from build123d import *

# Parameters (mm, degrees)
BOSS_EXTRUDE1_DEPTH = 53.975
CUT_EXTRUDE1_DEPTH  = 140.411114894
CUT_EXTRUDE2_DEPTH  = 3.175
BOSS_EXTRUDE2_DEPTH = 15.875
CUT_EXTRUDE3_DEPTH  = 12.7
CHAMFER1_SIZE       = 1.651
CUT_EXTRUDE4_DEPTH  = 12.7
FILLET1_R           = 12.7
SKETCH9_R           = 6.35
CUT_EXTRUDE5_DEPTH  = 12.7
SKETCH10_R          = 9.525
CUT_EXTRUDE6_DEPTH  = 3.175
SKETCH11_R          = 13.97
BOSS_EXTRUDE3_DEPTH = 4.1275
SKETCH12_R          = 11.43
CUT_EXTRUDE7_DEPTH  = 124.457441957
SKETCH13_W          = 29.21
SKETCH13_H          = 6.35
BOSS_EXTRUDE4_DEPTH = 17.78
CUT_EXTRUDE8_DEPTH  = 131.033845412
FILLET3_R           = 1.905
FILLET4_R           = 1.27


with BuildPart() as part:
    # Sketch1 → Boss-Extrude1 (new, symmetric)
    with BuildSketch(Plane.XY):
        with BuildLine():
            Line((0, 0), (0, 12.7))
            Line((0, 12.7), (76.2, 12.7))
            Line((76.2, 12.7), (118.856216575, -29.956216575))
            Line((118.856216575, -29.956216575), (112.57003729, -36.24239586))
            Line((112.57003729, -36.24239586), (91.206616946, -14.878975516))
            ThreePointArc((91.206616946, -14.878975516), (74.725910826, -3.866919748), (55.285592462, 0))
            Line((55.285592462, 0), (0, 0))
        make_face()
    extrude(amount=BOSS_EXTRUDE1_DEPTH, both=True)

    # Sketch2 → Cut-Extrude1 (cut, through all)
    with BuildSketch(Plane(origin=(0, 12.7, 0), x_dir=(1, 0, 0), z_dir=(0, 1, 0))):
        with BuildLine():
            Line((25.4, 53.975), (25.4, 34.925))
            ThreePointArc((25.4, 34.925), (38.1, 22.225), (50.8, 34.925))
            Line((50.8, 34.925), (50.8, 53.975))
            Line((50.8, 53.975), (25.4, 53.975))
        make_face()
        with BuildLine():
            Line((25.4, -53.975), (50.8, -53.975))
            Line((50.8, -53.975), (50.8, -34.925))
            ThreePointArc((50.8, -34.925), (38.1, -22.225), (25.4, -34.925))
            Line((25.4, -34.925), (25.4, -53.975))
        make_face()
    extrude(amount=-CUT_EXTRUDE1_DEPTH, mode=Mode.SUBTRACT)

    # Sketch4 → Cut-Extrude2 (cut, symmetric)
    with BuildSketch(Plane(origin=(0, 6.35, 0), x_dir=(1, 0, 0), z_dir=(0, 1, 0))):
        with BuildLine():
            Line((59.055, -34.925), (59.055, -53.975))
            Line((59.055, -53.975), (17.145, -53.975))
            Line((17.145, -53.975), (17.145, -34.925))
            ThreePointArc((17.145, -34.925), (38.1, -13.97), (59.055, -34.925))
        make_face()
        with BuildLine():
            Line((17.145, 53.975), (17.145, 34.925))
            ThreePointArc((17.145, 34.925), (38.1, 13.97), (59.055, 34.925))
            Line((59.055, 34.925), (59.055, 53.975))
            Line((59.055, 53.975), (17.145, 53.975))
        make_face()
    extrude(amount=CUT_EXTRUDE2_DEPTH, both=True, mode=Mode.SUBTRACT)

    # Sketch5 → Boss-Extrude2 (add, symmetric)
    with BuildSketch(Plane.XY):
        Polygon((0, 12.7), (0, 46.784531851), (76.2, 19.05), (76.2, 12.7), align=None)
    extrude(amount=BOSS_EXTRUDE2_DEPTH, both=True)

    # Sketch6 → Cut-Extrude3 (cut)
    with BuildSketch(Plane(origin=(15.036258699, 41.31178125, 0), x_dir=(0.9396926207859106, -0.3420201433256628, 0), z_dir=(0.3420201433256627, 0.9396926207859105, 0))):
        with BuildLine():
            Line((13.631742372, 3.175), (30.56575305, 3.175))
            ThreePointArc((30.56575305, 3.175), (52.197747711, 0), (30.56575305, -3.175))
            Line((30.56575305, -3.175), (13.631742372, -3.175))
            ThreePointArc((13.631742372, -3.175), (-8.000252289, 0), (13.631742372, 3.175))
        make_face()
    extrude(amount=-CUT_EXTRUDE3_DEPTH, mode=Mode.SUBTRACT)

    # Chamfer1
    chamfer1_edges = [part.edges().sort_by_distance(p)[0] for p in [
        (7.518480659, 44.048028684, 0),
        (35.802288852, 33.75356439, 3.175),
        (64.086097045, 23.459100096, 0),
        (35.802288852, 33.75356439, -3.175),
    ]]
    chamfer(chamfer1_edges, length=CHAMFER1_SIZE)

    # Sketch7 → Cut-Extrude4 (cut)
    with BuildSketch(Plane(origin=(44.45, 44.45, 0), x_dir=(0, 0, -1), z_dir=(0.7071067811865483, 0.7071067811865468, 0))):
        with BuildLine():
            Line((-34.925, -60.776280605), (-53.975, -60.776280605))
            Line((-53.975, -60.776280605), (-53.975, -105.226280605))
            Line((-53.975, -105.226280605), (-8.3e-08, -105.226280605))
            ThreePointArc((-8.3e-08, -105.226280605), (-11.225320181, -100.576600727), (-15.875, -89.351280605))
            Line((-15.875, -89.351280605), (-34.925, -89.351280605))
            Line((-34.925, -89.351280605), (-34.925, -60.776280605))
        make_face()
        with BuildLine():
            ThreePointArc((15.875, -89.351280605), (11.225320122, -100.576600786), (-8.3e-08, -105.226280605))
            Line((-8.3e-08, -105.226280605), (53.975, -105.226280605))
            Line((53.975, -105.226280605), (53.975, -60.776280605))
            Line((53.975, -60.776280605), (34.925, -60.776280605))
            Line((34.925, -60.776280605), (34.925, -89.351280605))
            Line((34.925, -89.351280605), (15.875, -89.351280605))
        make_face()
    extrude(amount=-CUT_EXTRUDE4_DEPTH, mode=Mode.SUBTRACT)

    # Fillet1
    fillet1_edges = [part.edges().sort_by_distance(p)[0] for p in [
        (104.487806781, -21.873986066, 34.925),
        (104.487806781, -21.873986066, -34.925),
        (0, 6.35, 53.975),
        (0, 6.35, -53.975),
    ]]
    fillet(fillet1_edges, radius=FILLET1_R)

    # Sketch9 → Cut-Extrude5 (cut)
    with BuildSketch(Plane(origin=(44.45, 44.45, 0), x_dir=(0, 0, -1), z_dir=(0.7071067811865482, 0.7071067811865468, 0))):
        with Locations(Location((-22.225, -76.651280605, 0), (0, 0, 90))):
            Circle(SKETCH9_R)
        with Locations(Location((22.225, -76.651280605, 0), (0, 0, 90))):
            Circle(SKETCH9_R)
    extrude(amount=-CUT_EXTRUDE5_DEPTH, mode=Mode.SUBTRACT)

    # Sketch10 → Cut-Extrude6 (cut)
    with BuildSketch(Plane(origin=(44.45, 44.45, 0), x_dir=(0, 0, -1), z_dir=(0.7071067811865482, 0.7071067811865468, 0))):
        with Locations(Location((-22.225, -76.651280605, 0), (0, 0, 90))):
            Circle(SKETCH10_R)
        with Locations(Location((22.225, -76.651280605, 0), (0, 0, 90))):
            Circle(SKETCH10_R)
    extrude(amount=-CUT_EXTRUDE6_DEPTH, mode=Mode.SUBTRACT)

    # Sketch11 → Boss-Extrude3 (add, symmetric)
    with BuildSketch(Plane(origin=(44.45, 44.45, 0), x_dir=(0, 0, -1), z_dir=(0.7071067811865482, 0.7071067811865468, 0))):
        with Locations(Location((0, -89.351280605, 0), (0, 0, 270))):
            Circle(SKETCH11_R)
    extrude(amount=BOSS_EXTRUDE3_DEPTH, both=True)

    # Sketch12 → Cut-Extrude7 (cut, through all)
    with BuildSketch(Plane(origin=(47.368583239, 47.368583239, 0), x_dir=(0, 0, -1), z_dir=(0.7071067811865483, 0.7071067811865468, 0))):
        with Locations(Location((0, -89.351280605, 0), (0, 0, 90))):
            Circle(SKETCH12_R)
    extrude(amount=-CUT_EXTRUDE7_DEPTH, mode=Mode.SUBTRACT)

    # Sketch13 → Boss-Extrude4 (add)
    with BuildSketch(Plane(origin=(44.45, 44.45, 0), x_dir=(0, 0, -1), z_dir=(0.7071067811865482, 0.7071067811865468, 0))):
        with Locations((-33.274, -52.838780605)):
            Rectangle(SKETCH13_W, SKETCH13_H)
        with Locations((33.274, -52.838780605)):
            Rectangle(SKETCH13_W, SKETCH13_H)
    extrude(amount=BOSS_EXTRUDE4_DEPTH)

    # Sketch14 → Cut-Extrude8 (cut, through all)
    with BuildSketch(Plane(origin=(39.607724106, -39.607724106, 0), x_dir=(0, 0, -1), z_dir=(0.7071067811865468, -0.7071067811865483, 0))):
        with BuildLine():
            ThreePointArc((-33.274, 80.641792847), (-22.946705461, 76.364087387), (-18.669, 66.036792847))
            Line((-18.669, 66.036792847), (-18.669, 80.641792847))
            Line((-18.669, 80.641792847), (-33.274, 80.641792847))
        make_face()
        with BuildLine():
            Line((-47.879, 80.641792847), (-47.879, 66.036792847))
            ThreePointArc((-47.879, 66.036792847), (-43.601294539, 76.364087387), (-33.274, 80.641792847))
            Line((-33.274, 80.641792847), (-47.879, 80.641792847))
        make_face()
        with BuildLine():
            Line((-44.704, 66.036792847), (-21.844, 66.036792847))
            ThreePointArc((-21.844, 66.036792847), (-33.274, 77.466792847), (-44.704, 66.036792847))
        make_face()
        with BuildLine():
            Line((18.669, 80.641792847), (18.669, 66.036792847))
            ThreePointArc((18.669, 66.036792847), (22.946705461, 76.364087387), (33.274, 80.641792847))
            Line((33.274, 80.641792847), (18.669, 80.641792847))
        make_face()
        with BuildLine():
            Line((47.879, 80.641792847), (33.274, 80.641792847))
            ThreePointArc((33.274, 80.641792847), (43.601294539, 76.364087387), (47.879, 66.036792847))
            Line((47.879, 66.036792847), (47.879, 80.641792847))
        make_face()
        with BuildLine():
            ThreePointArc((21.844, 66.036792847), (33.274, 77.466792847), (44.704, 66.036792847))
            Line((44.704, 66.036792847), (21.844, 66.036792847))
        make_face()
    extrude(amount=-CUT_EXTRUDE8_DEPTH, mode=Mode.SUBTRACT)

    # Fillet3
    fillet3_edges = [part.edges().sort_by_distance(p)[0] for p in [
        (84.057724106, 9.332403955, -21.844),
        (84.057724106, 9.332403955, -44.704),
        (84.057724106, 9.332403955, 21.844),
        (84.057724106, 9.332403955, 44.704),
    ]]
    fillet(fillet3_edges, radius=FILLET3_R)

    # Fillet4
    fillet4_edges = [part.edges().sort_by_distance(p)[0] for p in [
        (81.812660076, 7.087339924, 18.669),
        (79.567596045, 9.332403955, 33.274),
        (81.812660076, 7.087339924, 47.879),
        (84.057724106, 4.842275894, 33.274),
        (81.812660076, 7.087339924, -47.879),
        (79.567596045, 9.332403955, -33.274),
        (81.812660076, 7.087339924, -18.669),
        (84.057724106, 4.842275894, -33.274),
        (85.180256121, 5.964807909, 18.669),
        (80.690128061, 10.45493597, 18.669),
        (85.180256121, 5.964807909, -47.879),
        (80.690128061, 10.45493597, -47.879),
        (96.630082675, 17.414634464, 33.274),
        (92.139954615, 21.904762524, 33.274),
        (92.139954615, 21.904762524, -33.274),
        (96.630082675, 17.414634464, -33.274),
        (85.180256121, 5.964807909, 47.879),
        (80.690128061, 10.45493597, 47.879),
        (85.180256121, 5.964807909, -18.669),
        (80.690128061, 10.45493597, -18.669),
    ]]
    fillet(fillet4_edges, radius=FILLET4_R)


solid = part.part
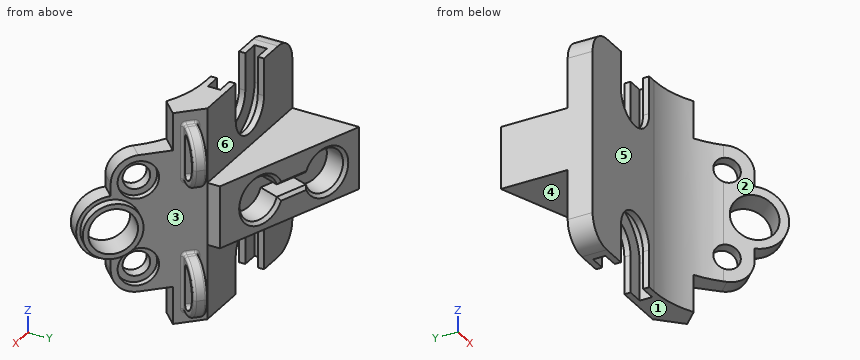
Input: part model. Units: mm. Frame: model coordinates. Face numbers are marked on the shaded views. A direction names the side the tool comes from. Coordinates: 2 decimals unless noted, no trailing zeros.
Q1. Contact query for flat-ended pins moving along their axis: pin 1 (5 mm diameter, centred on x = 77, z = -3.5, fed in from +Y); pin 2 (2 mm diameter, centred on y = 16.5, z = -19.5, fed in from +X); pin 3 (1.9 mm diameter, centred on y = 6.5, z = 47, fed in from -X); pin 4 (7 mm diameter, centred on y = 5.5, z = 43, fed in from +X). Output: stop coordinate, or through.
Q2. Cut plane A-A (z = -36.5). Give the number of separate pieces and of enclosed holes in the cut face, then the cut area to 3 significant figures.
Q3. Material intervals for line 1 (Y direction, x = 53.5, z = 31) (3 decimals); line 2 (Z direction, x = 106.5, y = -28.5); line 3 (Z direction, x = 38, y = 2), sorted ascending.
Q4. Draft query along Y for the marked faces 1, 2 and 3. Return one class per face: +Y half, -Y half, draft (parallel to the pull), parting line (faces both ways), or undercut.
Q5. Set-up query: the marked faces 4, 5 and 6. Return all of +Z, -Z, +X, -X, +Y, -Y with unobstructed straight access to the full face (end or side cutting, diameter ignored); none if empty.
Working result:
1. pin 1: stops at y = 19.67
1. pin 2: passes through
1. pin 3: stops at x = 0.93
1. pin 4: stops at x = 87.89
2. separate pieces: 3
2. enclosed holes: 0
2. area: 729 mm2
3. line 1: y = 0 to 3.175, 9.525 to 12.7
3. line 2: z = -14.65 to -9.66, 9.66 to 14.65
3. line 3: z = -22.23 to 22.23
4. face 1: draft
4. face 2: -Y half
4. face 3: undercut
5. face 4: -Z, +X, -X, +Y
5. face 5: +Z, -Z, -X, -Y
5. face 6: +Z, -X, +Y
